Geometry: final body of the model. Coordinates: model frame, mm. Round coordinates to 2 decimals unless told otherwise and drop trailing zeros. Loops run counter-clockwise (first coordinate to the right, second up) from the corner with the lowest first, then second, coordinate; pieces in that order, holes last. Notation, with made-up numbers: (46, 34.25) - (105, 34.25) arc R20 cw to (105, 64.25) - close; hole circle Ø5 at (68, 83). An arc over 180 degrees is marked (long way). Return JSON: item names as keys, results as strings. Group by question number.
1. Section C-C on y = -7.5. Return loops of the section in (x, z) (3 decimals), and give its area (3 significant figures).
2. First-contact query: pin 1 Ø4 at (x, y) = (34.5, 8) entering from -Z; pin 2 Ø6 at (x, y) = (11, -10.5) entering from -Z. Flat tips, straight axial feed; report the tip coordinate or a pass-through.
3. Section A-A on x = 2. Return loops of the section in (y, z).
4. Section B-B on z = 0.4. Return loops of the section in (x, y) (1 decimal).
5. Material intervals for probe 1 along X at (y, z) = (2, 1) (3 decimals); probe 2 along Y at (x, z) = (-37, 0.9); probe 3 along X at (y, z) = (-13.5, 2), sorted ascending.
from build123d import *

# Parameters (mm, degrees)
F0_W     = 16.51
F0_H     = 34.29
F0_W_2   = 33.02
F0_W_3   = 15.875
F1_DEPTH = 2.159
F2_R     = 1.016


with BuildPart() as f1:
    # F0 (on Top) → F1 (new body)
    with BuildSketch(Plane.XY):
        Polygon((-67.31, -10.4775), (-67.31, -24.4475), (-33.655, -24.4475), (0, -24.4475), (33.02, -24.4475), (67.31, -24.4475), (67.31, 0), (67.31, 24.4475), (33.02, 24.4475), (0, 24.4475), (-33.655, 24.4475), (-67.31, 24.4475), (-67.31, 10.4775), align=None)
        with Locations((-41.91, 0.635)):
            Rectangle(F0_W, F0_H, mode=Mode.SUBTRACT)
        with Locations((-0.635, 0.635)):
            Rectangle(F0_W_2, F0_H, mode=Mode.SUBTRACT)
        with Locations((40.9575, 0.635)):
            Rectangle(F0_W_3, F0_H, mode=Mode.SUBTRACT)
    extrude(amount=F1_DEPTH)

    # F2
    f2_edges = [f1.edges().sort_by_distance(p)[0] for p in [
        (15.875, 0.635, 2.159),
        (-33.655, 0.635, 2.159),
        (-17.145, 0.635, 2.159),
        (-50.165, 0.635, 2.159),
        (-41.91, 17.78, 2.159),
        (-0.635, 17.78, 2.159),
        (-0.635, -16.51, 2.159),
        (-41.91, -16.51, 2.159),
        (40.9575, -16.51, 2.159),
        (33.02, 0.635, 2.159),
        (40.9575, 17.78, 2.159),
        (48.895, 0.635, 2.159),
        (0, -24.4475, 2.159),
        (0, 24.4475, 2.159),
        (67.31, 0, 2.159),
    ]]
    fillet(f2_edges, radius=F2_R)


solid = f1.part
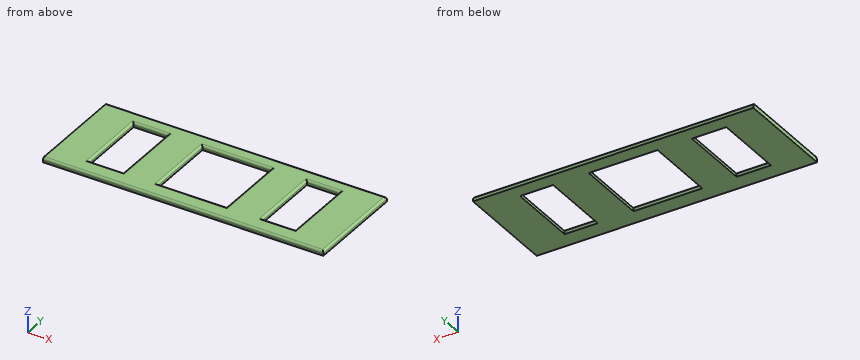
Taken from the geometry:
{
 "1": {"outline": "(-67.31, 0) - (-50.165, 0) - (-50.165, 1.143) arc R1.016 ccw to (-51.181, 2.159) - (-67.31, 2.159) - close; (-33.655, 0) - (-17.145, 0) - (-17.145, 1.143) arc R1.016 ccw to (-18.161, 2.159) - (-32.639, 2.159) arc R1.016 ccw to (-33.655, 1.143) - close; (15.875, 0) - (33.02, 0) - (33.02, 1.143) arc R1.016 ccw to (32.004, 2.159) - (16.891, 2.159) arc R1.016 ccw to (15.875, 1.143) - close; (48.895, 0) - (67.31, 0) - (67.31, 1.143) arc R1.016 ccw to (66.294, 2.159) - (49.911, 2.159) arc R1.016 ccw to (48.895, 1.143) - close", "area": "148 mm2"},
 "2": {"pin 1": "z = 0", "pin 2": "through"},
 "3": {"outline": "(-24.45, 0) - (-16.51, 0) - (-16.51, 1.14) arc R1.02 ccw to (-17.53, 2.16) - (-23.43, 2.16) arc R1.02 ccw to (-24.45, 1.14) - close; (17.78, 0) - (24.45, 0) - (24.45, 1.14) arc R1.02 ccw to (23.43, 2.16) - (18.8, 2.16) arc R1.02 ccw to (17.78, 1.14) - close"},
 "4": {"outline": "(-67.3, -24.4) - (67.3, -24.4) - (67.3, 24.4) - (-67.3, 24.4) - close; hole (-50.2, -16.5) - (-33.7, -16.5) - (-33.7, 17.8) - (-50.2, 17.8) - close; hole (-17.1, -16.5) - (15.9, -16.5) - (15.9, 17.8) - (-17.1, 17.8) - close; hole (33, -16.5) - (48.9, -16.5) - (48.9, 17.8) - (33, 17.8) - close"},
 "5": {"probe 1": "-67.31 to -50.165, -33.655 to -17.145, 15.875 to 33.02, 48.895 to 67.31", "probe 2": "-24.45 to -16.51, 17.78 to 24.45", "probe 3": "-67.31 to -50.64, -33.18 to -17.62, 16.35 to 32.55, 49.37 to 66.84"}
}
